```python
from build123d import *

# Parameters (mm, degrees)
EXTRUDE_1_DEPTH     = 40
CUT_EXTRUDE_1_REACH = 122
SKETCH_5_R          = 11
SKETCH_6_R          = 2
CUT_EXTRUDE_2_DEPTH = 20


with BuildPart() as part:
    # 草图1 → 凸台-拉伸1 (new body)
    with BuildSketch(Plane(origin=(0, 0, 0), x_dir=(0, 0, -1), z_dir=(1, 0, 0))):
        with BuildLine():
            Line((0, 0), (77, 0))
            ThreePointArc((77, 0), (82.656854249, 2.343145751), (85, 8))
            Line((85, 8), (85, 112))
            ThreePointArc((85, 112), (82.656854249, 117.656854249), (77, 120))
            Line((77, 120), (0, 120))
            Line((0, 120), (0, 110))
            Line((0, 110), (67, 110))
            ThreePointArc((67, 110), (72.656854249, 107.656854249), (75, 102))
            Line((75, 102), (75, 18))
            ThreePointArc((75, 18), (72.656854249, 12.343145751), (67, 10))
            Line((67, 10), (0, 10))
            Line((0, 10), (0, 0))
        make_face()
    extrude(amount=EXTRUDE_1_DEPTH)

    # 草图5 → 切除-拉伸1 (cut, up to next)
    with BuildSketch(Plane.XZ, mode=Mode.PRIVATE) as cut_extrude_1_sk1:
        with Locations((20, -35)):
            Circle(SKETCH_5_R)
    cut_extrude_1_tool1 = extrude(cut_extrude_1_sk1.sketch, amount=-CUT_EXTRUDE_1_REACH, mode=Mode.PRIVATE) & part.part
    add(cut_extrude_1_tool1.solids().sort_by_distance((20, 0, -35))[0], mode=Mode.SUBTRACT)

    # 草图6 → 切除-拉伸2 (cut)
    with BuildSketch(Plane.XZ):
        with Locations((8, -10)):
            Circle(SKETCH_6_R)
        with Locations((32, -10)):
            Circle(SKETCH_6_R)
        with Locations((8, -60)):
            Circle(SKETCH_6_R)
        with Locations((32, -60)):
            Circle(SKETCH_6_R)
    extrude(amount=-CUT_EXTRUDE_2_DEPTH, mode=Mode.SUBTRACT)


solid = part.part
```
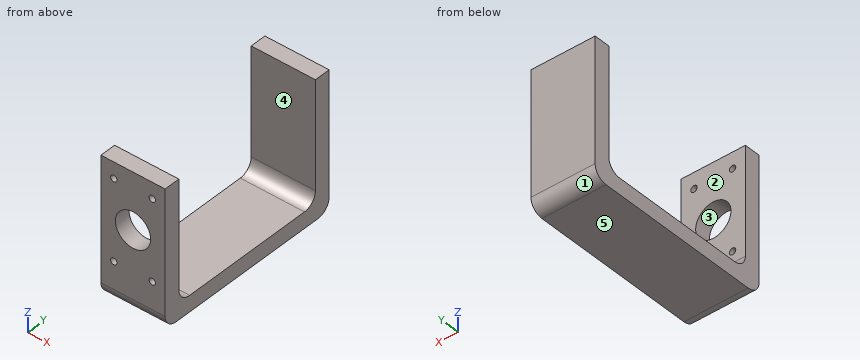
CAD build for the part. Positions are in the model's coordinates, mm. Face numbers are marked on the shaded views. A direction names the side the tool comes from. Give positions to 0.01 mm unless a question says otherwise; leave off trailing zeros. Order: outer loops, then holes, each group sorted by start corner. A loop starts at its lowest first (then second) coordinate and runs counter-clockwise, first axis right, second up.
(1) Saw through at C-C, the plane z = -60. Give the cut face in (x, y), then the cut area to 3 significant figures.
(2) Mould opens along Y. For the marked faces 1, 2 and 3 say: released by +Y, released by -Y, zero draft, split by the parting line, or undercut.
(3) Drill centre lines: L1, parallel to Z at x = 32, y = 4; L2, parallel to Z at x = 8, y = 4.75; L3, parallel to Y at x = 18, z = -65. Where is each one in solid material? Low to high.
(4) Flat gauge pins, fed straight in: pin 1 (12 mm diameter, centred on x = 15, y = 41.5, fed in from +Z); pin 2 (13 mm diameter, centred on x = 20, z = -35, fed in from -Y). Where does each tip first touch, or does it go through?
(5) Tool access for the marked faces 4 and 5: list every direction of +Z, -Z, +X, -X, +Y, -Y with a clear straight run to the whole face (end or side of a thin tool).
(6) Saw through at B-B, the plane z = -50. Give the cut face in (x, y), then the cut area to 3 significant figures.
(7) Saw through at A-A, the plane x = 20. Give the cut face in (y, z), then the cut area to 3 significant figures.
(8) Saw through at D-D, the plane y = 41. Give the cut face in (x, z).
Results found:
1. outline: (0, 0) - (6, 0) - (6, 10) - (0, 10) - close; (0, 110) - (40, 110) - (40, 120) - (0, 120) - close; (10, 0) - (30, 0) - (30, 10) - (10, 10) - close; (34, 0) - (40, 0) - (40, 10) - (34, 10) - close
1. area: 720 mm2
2. face 1: released by +Y
2. face 2: undercut
2. face 3: zero draft
3. L1: z = -83.93 to -62, -58 to -12, -8 to 0
3. L2: z = -84.31 to -62, -58 to -12, -8 to 0
3. L3: y = 0 to 10, 110 to 120
4. pin 1: stops at z = -75
4. pin 2: stops at y = 110
5. face 4: +Z, +X, -X
5. face 5: -Z, +X, -X, +Y, -Y
6. outline: (0, 0) - (40, 0) - (40, 10) - (0, 10) - close; (0, 110) - (40, 110) - (40, 120) - (0, 120) - close
6. area: 800 mm2
7. outline: (0, -77) arc R8 ccw to (8, -85) - (112, -85) arc R8 ccw to (120, -77) - (120, 0) - (110, 0) - (110, -67) arc R8 cw to (102, -75) - (18, -75) arc R8 cw to (10, -67) - (10, -46) - (0, -46) - close; (0, -24) - (10, -24) - (10, 0) - (0, 0) - close
7. area: 2,480 mm2
8. outline: (0, -85) - (40, -85) - (40, -75) - (0, -75) - close
